Autodesk Inventor part; units mm, degrees
ref_plane "Work Plane1" through (0, 0, 30) normal (0, 0, 1) x (1, 0, 0)
ref_plane "YZ Plane" through (0, 0, 0) normal (1, 0, 0) x (0, 1, 0)
ref_plane "XZ Plane" through (0, 0, 0) normal (0, 1, 0) x (-1, 0, 0)
sketch "Sketch1" plane through (0, 0, 0) normal (0, 0, 1) x (1, 0, 0)
  line L0 (0, 0) -> (575, 0)
  line L1 (575, 0) -> (575, 30)
  line L2 (575, 30) -> (200, 22)
  line L3 (200, 22) -> (0, 22)
  line L4 (0, 22) -> (0, 0)
  dimension "d0" = 575
  dimension "d1" = 30
  dimension "d2" = 22
  dimension "d3" = 200
revolve "Revolution1" add sketch "Sketch1" angle 360 about axis through (0, 0, 0) along (1, 0, 0)
ref_plane "Work Plane1" through (0, 0, 30) normal (0, 0, 1) x (1, 0, 0)
sketch "Sketch2" plane through (0, 0, 30) normal (0, 0, 1) x (1, 0, 0)
  line L0 (515, 39.8306) -> (599.6476, 39.8306)
  line L1 (599.6476, 39.8306) -> (599.6476, 10)
  line L2 (599.6476, 10) -> (515, 10)
  line L3 (515, 10) -> (515, 39.8306)
  line L4 (509.4984, 0) -> (515, 0)
  line L5 (575, -30) -> (575, 30)
  line L6 (512.2492, 0) -> (602.6525, 0)
  line L7 (515, -39.8306) -> (599.6476, -39.8306)
  line L8 (599.6476, -39.8306) -> (599.6476, -10)
  line L9 (599.6476, -10) -> (515, -10)
  line L10 (515, -10) -> (515, -39.8306)
  point P0 (0, 0)
  dimension "d6" = 60
  dimension "d7" = 10
extrude "Extrusion1" cut sketch "Sketch2" along normal through all both and the other way through all
sketch "Sketch3" plane through (575, 10, 28.2843) normal (0, 1, 0) x (1, 0, 0)
  line L0 (-60, 55.2071) -> (-60, 1.3614)
  line L1 (-60, 55.2071) -> (-28.0755, 55.2071)
  line L2 (-28.0755, 2.2843) -> (-60, 2.2843)
  line L3 (-60, 55.2071) -> (-60, 2.2843)
  arc A0 (-28.0755, 2.2843) -> (-28.0755, 55.2071) centre (-28.0755, 28.7457) ccw
  line L4 (-60, 65.181) -> (5.1582, 65.181)
  line L5 (5.1582, 65.181) -> (5.1582, -12.094)
  line L6 (5.1582, -12.094) -> (-60, -12.094)
  line L7 (-60, -12.094) -> (-60, 65.181)
  point P0 (-575, 28.2843)
  point P1 (-60, 1.3614)
extrude "Extrusion2" cut sketch "Sketch3" along normal through all both and the other way through all contours L7 L4 L5 L6 L0 L2 A0 L1
sketch "Sketch4" plane through (515, 10, -26.9228) normal (0, 1, 0) x (1, 0, 0)
  circle A0 centre (31.9245, -26.9228) radius 9.5
  point P0 (-515, -26.9228)
  dimension "d12" = 19
extrude "Extrusion3" cut sketch "Sketch4" against normal through all
mirror "Mirror1" about plane through (0, 0, 0) normal (1, 0, 0) of "Revolution1", "Extrusion2", "Extrusion3", "Extrusion1"
properties part number "Arjun_SteeringRod"
Geometry: final body of the model. Coordinates: model frame, mm. A direction names the side the tool comes from. Round coordinates to 2 decimals unless told otherwise and drop trailing zeros. Order: outer loops, then holes, each group sorted by start corner. A loop starts at its lowest first (then second) coordinate and runs counter-clockwise, first axis right, second up. Notation, with made-up numbers: M 25,70.25 L 44,70.25 A15 ccw 44,91.25 Z; hole C 4.25,9 d7. An arc over 180 degrees is marked long. Use one line per item in the form item = value. Start each with the question number.
Q1. Pin query (flat end, axial travel): pin 1 Ø5 at (x, z) = (29, 5.5) entering from +Y; pin 2 Ø12 at (x, y) = (189.5, -21.5) entering from -Z; pin 3 Ø10 at (x, z) = (55, -1.5) entering from -Y. Return the tip coordinate at first contact, or that it passes through.
Q2. Access query for faces 1 (the face through (-359.705, 24.234, -7.632)), 2 (the face through (-537, 10, 0)), 3 (the face through (-537, -10, 0)), 4 (the face through (531, 0, -26.923)). Directions: +Z, -Z, +X, -X, +Y, -Y. A direction counts if a zero-diameter tool reaches every point of the face in a straight line with its end or side. Return the directions, or none.
Q3. Cut plane A-A (y = 0). Return loops of the section in (x, z).
Q4. Cut plane D-D (x = -424). Return loops of the section in (y, z), and give its area (3 significant figures).
Q5. Mould query, pull axis Z, two halves, no side actions, for faces 5 (the face through (538, -10, -6)), 6 (the face through (531, 0, 26)), 7 (the face through (555.986, 0.14, -2.854)). Classes: +Z half, -Z half, draft (parallel to the pull), parting line (faces both ways), or undercut.
Q6. Cut plane C-C (x = 69). Return loops of the section in (y, z).
Q7. Material intervals for line 1 (X direction, y = 3.5, z = -2); line 2 (X direction, y = -5, z = 0); line 3 (Y direction, x = 524.5, z = 1), sorted ascending. Write a range as [from, to].
Q8. Cut plane B-B (z = 0). Return loops of the section in (x, y), and give its area (3 significant figures).
Geometry results:
q1.pin_1 = 21.79
q1.pin_2 = -15.61
q1.pin_3 = -22
q2.face_1 = none
q2.face_2 = +Z, -Z, -X, +Y
q2.face_3 = +Z, -Z, -X, -Y
q2.face_4 = -Z, +X, +Y, -Y
q3.outline = M -546.92,-26.92 L -515,-26.92 L -515,-28.72 L -200,-22 L 200,-22 L 515,-28.72 L 515,-26.92 L 546.92,-26.92 A26.46 ccw 546.92,26 L 515,26 L 515,28.72 L 200,22 L -200,22 L -515,28.72 L -515,26 L -546.92,26 A26.46 ccw Z; hole C -546.92,0 d19; hole C 546.92,0 d19
q4.outline = C 0,0 d53.56
q4.area = 2,250 mm^2
q5.face_5 = draft
q5.face_6 = +Z half
q5.face_7 = undercut
q6.outline = C 0,0 d44
q7.line_1 = [-573.34, -556.21], [-537.64, 537.64], [556.21, 573.34]
q7.line_2 = [-573.38, -556.42], [-537.42, 537.42], [556.42, 573.38]
q7.line_3 = [-10, 10]
q8.outline = M -573.38,-10 L -556.42,-10 L -556.42,10 L -573.38,10 Z; M -537.42,-10 L -515,-10 L -515,-28.72 L -200,-22 L 200,-22 L 515,-28.72 L 515,-10 L 537.42,-10 L 537.42,10 L 515,10 L 515,28.72 L 200,22 L -200,22 L -515,28.72 L -515,10 L -537.42,10 Z; M 556.42,-10 L 573.38,-10 L 573.38,10 L 556.42,10 Z
q8.area = 51,100 mm^2
